Model file for the job. Use its own axes, mm. A direction names the side the tool comes from. Round coordinates to 2 decimals unless told otherwise and drop trailing zeros. Loops run counter-clockwise (first coordinate to the right, second up) from the corner with the lowest first, then second, coordinate; pieces in that order, holes last. Notation, with made-up numbers: (30.25, 64) -> (89.25, 64) arc R28 ccw to (89.25, 93) -> close; hole circle Ø11 at (-11, 43). An arc over 180 degrees is marked (long way). Use a Markdown table: item, result. Add a question column.
```python
from build123d import *

# Parameters (mm, degrees)
RESSALTO_EXTRUS_O1_DEPTH  = 5
FILETE1_R                 = 10
ESBO_O4_R                 = 1.5
CORTE_EXTRUS_O3_DEPTH     = 124.512688994
ESPELHAR4_COPY_1_SKETCH_R = 1.5
ESPELHAR4_COPY_1_DEPTH    = 124.512688994
SKETCH1_W                 = 122
SKETCH1_H                 = 79
CUT_EXTRUDE1_DEPTH        = 124.512688994
FILLET2_R                 = 2
ESBO_O6_R                 = 1
CORTE_EXTRUS_O4_DEPTH     = 124.512688994
ESBO_O8_R                 = 1
ESBO_O8_R_2               = 1.042538076
CORTE_EXTRUS_O5_DEPTH     = 124.512688994
ESBO_O12_W                = 13
ESBO_O12_H                = 8.25
CORTE_EXTRUS_O7_DEPTH     = 124.512688994
ESBO_O13_R                = 1.5
CORTE_EXTRUS_O8_DEPTH     = 124.512688994
ESBO_O14_R                = 1
ESBO_O14_R_2              = 0.885907966
CORTE_EXTRUS_O9_DEPTH     = 124.512688994


with BuildPart() as part:
    # Esboço1 → Ressalto-extrusão1 (new body)
    with BuildSketch(Plane(origin=(0, 0, 0), x_dir=(1, 0, 0), z_dir=(0, 1, 0))):
        with BuildLine():
            Line((-69.062404082, -72.321396159), (69.062404082, -72.321396159))
            ThreePointArc((69.062404082, -72.321396159), (100, 0), (69.062404082, 72.321396159))
            Line((69.062404082, 72.321396159), (-69.062404082, 72.321396159))
            ThreePointArc((-69.062404082, 72.321396159), (-100, 0), (-69.062404082, -72.321396159))
        make_face()
    extrude(amount=RESSALTO_EXTRUS_O1_DEPTH)

    # Filete1
    filete1_edges = [part.edges().sort_by_distance(p)[0] for p in [
        (-69.062404082, 2.5, -72.321396159),
        (69.062404082, 2.5, -72.321396159),
        (69.062404082, 2.5, 72.321396159),
        (-69.062404082, 2.5, 72.321396159),
    ]]
    fillet(filete1_edges, radius=FILETE1_R)

    # Esboço4 → Corte-extrusão3 (cut, through all)
    with BuildSketch(Plane(origin=(0, 5, 0), x_dir=(1, 0, 0), z_dir=(0, 1, 0))):
        with Locations(Location((-50, 55, 0), (0, 0, 270))):
            Circle(ESBO_O4_R)
    corte_extrus_o3 = extrude(amount=-CORTE_EXTRUS_O3_DEPTH, mode=Mode.SUBTRACT)

    # Espelhar3: Corte-extrusão3 across plane
    add(corte_extrus_o3.mirror(Plane(origin=(0, 0, 0), x_dir=(0, 0, 1), z_dir=(1, 0, 0))), mode=Mode.SUBTRACT)

    # Espelhar4: Corte-extrusão3 across plane
    add(corte_extrus_o3.mirror(Plane.XY), mode=Mode.SUBTRACT)

    # Espelhar4 copy 1 sketch → Espelhar4 copy 1 (cut, through all)
    with BuildSketch(Plane(origin=(0, 5, 0), x_dir=(-1, 0, 0), z_dir=(0, 1, 0))):
        with Locations(Location((-50, 55, 0), (0, 0, 270))):
            Circle(ESPELHAR4_COPY_1_SKETCH_R)
    extrude(amount=-ESPELHAR4_COPY_1_DEPTH, mode=Mode.SUBTRACT)

    # Sketch1 → Cut-Extrude1 (cut, through all)
    with BuildSketch(Plane(origin=(0, 5, 0), x_dir=(1, 0, 0), z_dir=(0, 1, 0))):
        Rectangle(SKETCH1_W, SKETCH1_H)
    extrude(amount=-CUT_EXTRUDE1_DEPTH, mode=Mode.SUBTRACT)

    # Fillet2
    fillet2_edges = [part.edges().sort_by_distance(p)[0] for p in [
        (-61, 2.5, 39.5),
        (-61, 2.5, -39.5),
        (61, 2.5, -39.5),
        (61, 2.5, 39.5),
    ]]
    fillet(fillet2_edges, radius=FILLET2_R)

    # Esboço6 → Corte-extrusão4 (cut, through all)
    with BuildSketch(Plane(origin=(0, 5, 0), x_dir=(1, 0, 0), z_dir=(0, 1, 0))):
        with Locations(Location((-76.920436381, 19.236111974, 0), (0, 0, 270))):
            Circle(ESBO_O6_R)
        with Locations(Location((-76.920436293, -19.238117897, 0), (0, 0, 270))):
            Circle(ESBO_O6_R)
    extrude(amount=-CORTE_EXTRUS_O4_DEPTH, mode=Mode.SUBTRACT)

    # Esboço8 → Corte-extrusão5 (cut, through all)
    with BuildSketch(Plane(origin=(0, 5, 0), x_dir=(1, 0, 0), z_dir=(0, 1, 0))):
        with Locations(Location((76.920436129, -19.756156804, 0), (0, 0, 270))):
            Circle(ESBO_O8_R)
        with Locations(Location((76.920436041, 18.718073068, 0), (0, 0, 270))):
            Circle(ESBO_O8_R_2)
        with BuildLine():
            Line((77.058773716, -5.618000613), (68.478773716, -5.618000613))
            ThreePointArc((68.478773716, -5.618000613), (67.771666935, -5.325107395), (67.478773716, -4.618000613))
            Line((67.478773716, -4.618000613), (67.478773716, 4.381999387))
            ThreePointArc((67.478773716, 4.381999387), (67.771666935, 5.089106168), (68.478773716, 5.381999387))
            Line((68.478773716, 5.381999387), (77.058773716, 5.381999387))
            ThreePointArc((77.058773716, 5.381999387), (77.765880497, 5.089106168), (78.058773716, 4.381999387))
            Line((78.058773716, 4.381999387), (78.058773716, -4.618000613))
            ThreePointArc((78.058773716, -4.618000613), (77.765880497, -5.325107395), (77.058773716, -5.618000613))
        make_face()
    extrude(amount=-CORTE_EXTRUS_O5_DEPTH, mode=Mode.SUBTRACT)

    # Esboço12 → Corte-extrusão7 (cut, through all)
    with BuildSketch(Plane(origin=(0, 5, 0), x_dir=(1, 0, 0), z_dir=(0, 1, 0))):
        with Locations((-76.958855033, -37.107917316)):
            Rectangle(ESBO_O12_W, ESBO_O12_H)
        with BuildLine():
            Line((-77.058773716, 5.160452578), (-68.478773716, 5.160452578))
            ThreePointArc((-68.478773716, 5.160452578), (-67.771666935, 4.867559359), (-67.478773716, 4.160452578))
            Line((-67.478773716, 4.160452578), (-67.478773716, -4.839547422))
            ThreePointArc((-67.478773716, -4.839547422), (-67.771666935, -5.546654203), (-68.478773716, -5.839547422))
            Line((-68.478773716, -5.839547422), (-77.058773716, -5.839547422))
            ThreePointArc((-77.058773716, -5.839547422), (-77.765880497, -5.546654203), (-78.058773716, -4.839547422))
            Line((-78.058773716, -4.839547422), (-78.058773716, 4.160452578))
            ThreePointArc((-78.058773716, 4.160452578), (-77.765880497, 4.867559359), (-77.058773716, 5.160452578))
        make_face()
    extrude(amount=-CORTE_EXTRUS_O7_DEPTH, mode=Mode.SUBTRACT)

    # Esboço13 → Corte-extrusão8 (cut, through all)
    with BuildSketch(Plane(origin=(0, 5, 0), x_dir=(1, 0, 0), z_dir=(0, 1, 0))):
        with Locations(Location((-58, -55, 0), (0, 0, 270))):
            Circle(ESBO_O13_R)
        with Locations(Location((58, -55, 0), (0, 0, 90))):
            Circle(ESBO_O13_R)
        with Locations(Location((58, 55, 0), (0, 0, 270))):
            Circle(ESBO_O13_R)
        with Locations(Location((-58, 55, 0), (0, 0, 90))):
            Circle(ESBO_O13_R)
    extrude(amount=-CORTE_EXTRUS_O8_DEPTH, mode=Mode.SUBTRACT)

    # Esboço14 → Corte-extrusão9 (cut, through all)
    with BuildSketch(Plane(origin=(0, 5, 0), x_dir=(1, 0, 0), z_dir=(0, 1, 0))):
        with Locations(Location((-29.57071729, -58.018271029, 0), (0, 0, 270))):
            Circle(ESBO_O14_R)
        with Locations(Location((30.42928271, -58.018271029, 0), (0, 0, 270))):
            Circle(ESBO_O14_R_2)
        with BuildLine():
            Line((-14.930567591, -48.170190889), (-8.830173292, -48.170190889))
            ThreePointArc((-8.830173292, -48.170190889), (-8.123066511, -48.463084108), (-7.830173292, -49.170190889))
            Line((-7.830173292, -49.170190889), (-7.830173292, -57.018271029))
            ThreePointArc((-7.830173292, -57.018271029), (-8.123066511, -57.72537781), (-8.830173292, -58.018271029))
            Line((-8.830173292, -58.018271029), (-14.930567591, -58.018271029))
            ThreePointArc((-14.930567591, -58.018271029), (-15.637674372, -57.72537781), (-15.930567591, -57.018271029))
            Line((-15.930567591, -57.018271029), (-15.930567591, -49.170190889))
            ThreePointArc((-15.930567591, -49.170190889), (-15.637674372, -48.463084108), (-14.930567591, -48.170190889))
        make_face()
        with BuildLine():
            Line((9.546710766, -48.170190889), (15.764502084, -48.170190889))
            ThreePointArc((15.764502084, -48.170190889), (16.471608865, -48.463084108), (16.764502084, -49.170190889))
            Line((16.764502084, -49.170190889), (16.764502084, -57.018271029))
            ThreePointArc((16.764502084, -57.018271029), (16.471608865, -57.72537781), (15.764502084, -58.018271029))
            Line((15.764502084, -58.018271029), (9.546710766, -58.018271029))
            ThreePointArc((9.546710766, -58.018271029), (8.839603985, -57.72537781), (8.546710766, -57.018271029))
            Line((8.546710766, -57.018271029), (8.546710766, -49.170190889))
            ThreePointArc((8.546710766, -49.170190889), (8.839603985, -48.463084108), (9.546710766, -48.170190889))
        make_face()
    corte_extrus_o9 = extrude(amount=-CORTE_EXTRUS_O9_DEPTH, mode=Mode.SUBTRACT)

    # Espelhar5: Corte-extrusão9 across plane
    add(corte_extrus_o9.mirror(Plane.XY), mode=Mode.SUBTRACT)


solid = part.part
```
1) Cut at A-A on x = 43.5. Write the cut outline in (y, z).
2) Cut at C-C on y = 1.35. Count the separate pieces of the cut face and the enclosed holes in it, and give its area (3 significant figures).
3) Tool access for faces 4 (the face through (-15.931, 3, 53)), 5 (the face through (-1, 5, 47)): list every direction of +Z, -Z, +X, -X, +Y, -Y with a clear straight run to the whole face (end or side of a thin tool).
4) Cut at B-B on z = 13. Write the cut outline in (x, y), and give its area (3 significant figures).
5) Cut at D-D on z = -61. Write the cut outline in (x, y), and give its area (3 significant figures).
6) Pull direction Z, two halves, no side cores. Call faces 1 (the face through (-78.059, 3, 0)), 2 (the face through (-1, 0, 47)), 3 (the face through (68.8, 2.535, 71.542)): +Z half, -Z half, draft (parallel to the pull), parting line (faces both ways), or undercut.
7) Pin check, flat tips, straight feed: pin 1 Ø1.5 at (y, z) = (1.5, 52) entering from +X; pin 2 Ø4 at (x, z) = (50, 55) entering from +Y; pin 3 Ø1.6 at (x, z) = (-29.57, 58.02) entering from -Y; pin 4 Ø1 at (y, z) = (2.5, -13.5) entering from -X. Stop position of each tip, or through.
8) Wall check: probe 1 along Z at (x, y) = (10, 3.8); probe 2 along X at (y, z) = (1.9, -2); probe 3 along Z at (x, y) = (-4.5, 2.3). Give the ranges that are in metal, low to high. Write a range as from..to.
Established:
| question | item | result |
|---|---|---|
| 1 | outline | (0, -72.32) -> (5, -72.32) -> (5, -39.5) -> (0, -39.5) -> close; (0, 39.5) -> (5, 39.5) -> (5, 72.32) -> (0, 72.32) -> close |
| 2 | separate pieces | 1 |
| 2 | enclosed holes | 24 |
| 2 | area | 15,800 mm^2 |
| 3 | face 4 | +Y, -Y |
| 3 | face 5 | +Z, -Z, +X, -X, +Y |
| 4 | outline | (-99.15, 0) -> (-61, 0) -> (-61, 5) -> (-99.15, 5) -> close; (61, 0) -> (99.15, 0) -> (99.15, 5) -> (61, 5) -> close |
| 4 | area | 382 mm^2 |
| 5 | outline | (-79.24, 0) -> (79.24, 0) -> (79.24, 5) -> (-79.24, 5) -> close |
| 5 | area | 792 mm^2 |
| 6 | face 1 | undercut |
| 6 | face 2 | draft |
| 6 | face 3 | +Z half |
| 7 | pin 1 | stops at x = 85.87 |
| 7 | pin 2 | stops at y = 5 |
| 7 | pin 3 | passes through |
| 7 | pin 4 | stops at x = -99.15 |
| 8 | probe 1 | z = -72.32..-58.02, -48.17..-39.5, 39.5..48.17, 58.02..72.32 |
| 8 | probe 2 | x = -99.98..-78.06, -67.48..-61, 61..67.48, 78.06..99.98 |
| 8 | probe 3 | z = -72.32..-39.5, 39.5..72.32 |
